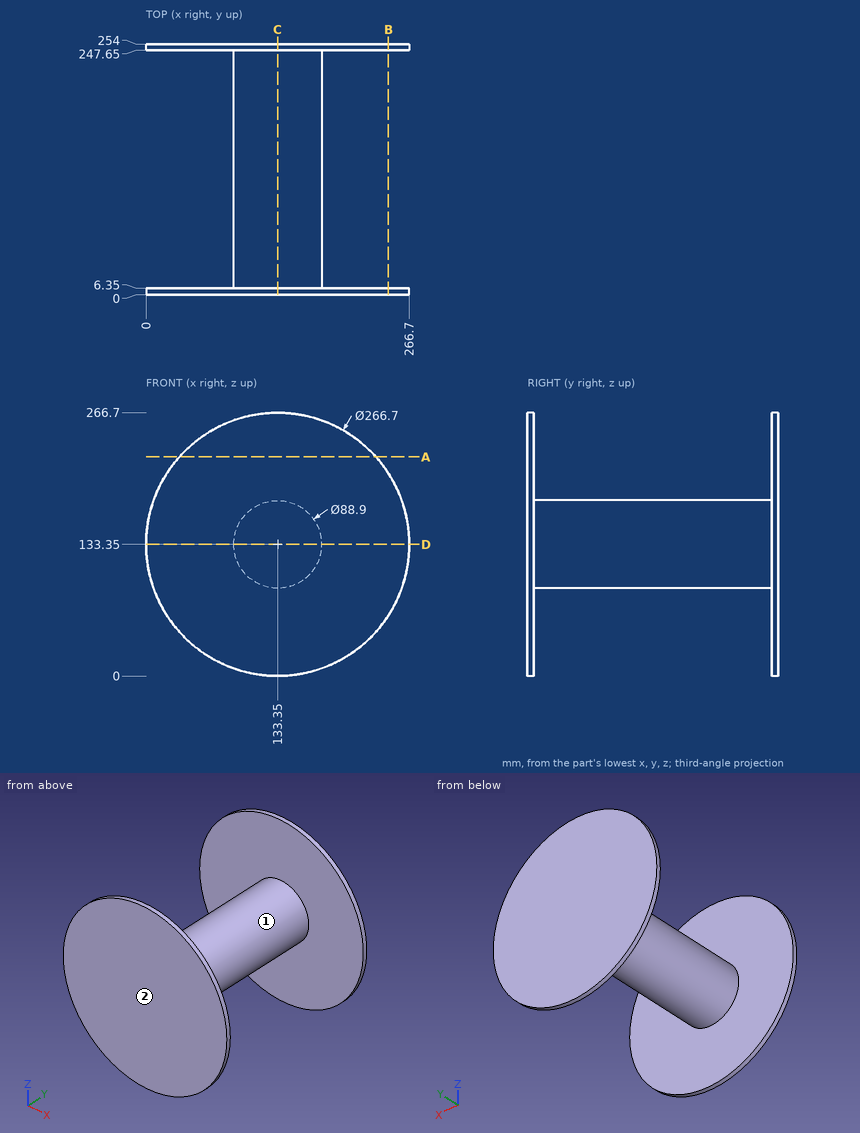
Check sheet for the drawn part. Datum: minimum x, y, z corner. Units: mm. A direction names the side the tool comes from. Give positions to 0.01 mm unless a question says otherwise; leave off trailing zeros. Order: outer loops, then holes, each group sorted by start corner. A loop starts at its lowest first (then second) coordinate and runs counter-clockwise, first axis right, second up. Notation, with made-up numbers: (63.25, 46.5) -> (79.25, 46.5) arc R21 ccw to (79.25, 55.5) -> close; hole circle Ø9 at (56.5, 51). An arc over 180 degrees is marked (long way). Use a Markdown table: item, result.
1) Section check A-A, the plane z = 222. Record the boundary of the cut face in (x, y), then the cut area to 3 significant figures.
Results:
| item | result |
|---|---|
| outline | (33.73, 0) -> (232.97, 0) -> (232.97, 6.35) -> (33.73, 6.35) -> close; (33.73, 247.65) -> (232.97, 247.65) -> (232.97, 254) -> (33.73, 254) -> close |
| area | 2,530 mm² |
2) Section check D-D, the plane z = 133.35. Record the boundary of the cut face in (x, y), then the cut area to 3 significant figures.
Results:
| item | result |
|---|---|
| outline | (0, 0) -> (266.7, 0) -> (266.7, 6.35) -> (177.8, 6.35) -> (177.8, 247.65) -> (266.7, 247.65) -> (266.7, 254) -> (0, 254) -> (0, 247.65) -> (88.9, 247.65) -> (88.9, 6.35) -> (0, 6.35) -> close |
| area | 24,800 mm² |
3) Tool access check on the marked faces 1 and 2. Record the directions out of +Z, -Z, +X, -X, +Y, -Y that give a thin tool (end or side, any length) a straight path to the whole face; none if there is none.
Results:
| item | result |
|---|---|
| face 1 | none |
| face 2 | +Z, -Z, +X, -X, -Y |
4) Material ranges on probe 1 along Y at (x, z) = (209, 229); probe 2 along X at (y, z) = (228, 133); probe 3 along X at (y, z) = (64.5, 126), recorded low to high.
Results:
| item | result |
|---|---|
| probe 1 | 0 to 6.35, 247.65 to 254 |
| probe 2 | 88.9 to 177.8 |
| probe 3 | 89.51 to 177.19 |
5) Section check C-C, the plane x = 133.35. Record the boundary of the cut face in (y, z), then the cut area to 3 significant figures.
Results:
| item | result |
|---|---|
| outline | (0, 0) -> (6.35, 0) -> (6.35, 88.9) -> (247.65, 88.9) -> (247.65, 0) -> (254, 0) -> (254, 266.7) -> (247.65, 266.7) -> (247.65, 177.8) -> (6.35, 177.8) -> (6.35, 266.7) -> (0, 266.7) -> close |
| area | 24,800 mm² |
6) Section check B-B, the plane x = 245.5. Record the boundary of the cut face in (y, z), then the cut area to 3 significant figures.
Results:
| item | result |
|---|---|
| outline | (0, 61.21) -> (6.35, 61.21) -> (6.35, 205.49) -> (0, 205.49) -> close; (247.65, 61.21) -> (254, 61.21) -> (254, 205.49) -> (247.65, 205.49) -> close |
| area | 1,830 mm² |
7) Depth check by flat-ended pin: pin 1 Ø6 at (x, y) = (100, 30) entering from +Z; pin 2 Ø1.5 at (x, y) = (96, 145.5) entering from -Z; pin 3 Ø12 at (x, y) = (110, 217) entering from +Z. Enter the tip coordinate at first touch or a pass-through.
Results:
| item | result |
|---|---|
| pin 1 | z = 165.83 |
| pin 2 | z = 108.13 |
| pin 3 | z = 174.27 |
